The drawing under review shows one solid part. Ordinate dimensions are in mm from its lowest x, y, z. A direction names the side the tool comes from. Coordinates: 2 decimals unless noted, no trailing zeros. Loops run counter-clockwise (first coordinate to the right, second up) from the corner with the lowest first, then second, coordinate; pieces in that order, holes last. Notation, with made-up numbers: (51.5, -1.5) - (57.5, -1.5) arc R11 cw to (57.5, 2.5) - close; hole circle Ø3 at (45.5, -14). An arc over 180 degrees is marked (long way). Answer as a JSON object with one key per item and string values. Group by question number.
Item 1: Clearance check with flat-ended pins moving along their axes: pin 1 (3 mm diameter, centred on x = 10.5, y = 11.5, fed in from +Z); pin 2 (4 mm diameter, centred on x = 18.5, y = 15, fed in from +Z); pin 3 (3 mm diameter, centred on x = 13.5, y = 14, fed in from +Z). State where each tip first meets the part, or that it passes through.
Item 2: We need section D-D (x = 17.5). Give the boundary of the cut face in (y, z).
Item 3: Tool access review of the marked faces 1 and 2: name each direction out of +Z, -Z, +X, -X, +Y, -Y from which nothing blocks a thin tool from reaching the whole face with its end or side.
Item 4: Mouldability with a two-part tool opening along X and no side actions: class the marked faces 3, 4 and 5 as released by +X, released by -X, zero draft, split by the parting line, or undercut.
Item 5: We need section C-C (y = 11). Give the boundary of the cut face in (x, z).
Item 6: We need section A-A (z = 11). Give the boundary of the cut face in (x, y).
Item 7: We need section B-B (x = 11.75). Give the boundary of the cut face in (y, z), then the cut area to 3 significant figures.
Item 8: To check wall thickness, follow line 1 (Y direction, x = 12.5, z = 1.9); line 2 (X direction, y = 14.75, z = 2.75); line 3 (Y direction, x = 10.75, z = 4.5). State the ranges of each line that lie inside material, in increasing order.
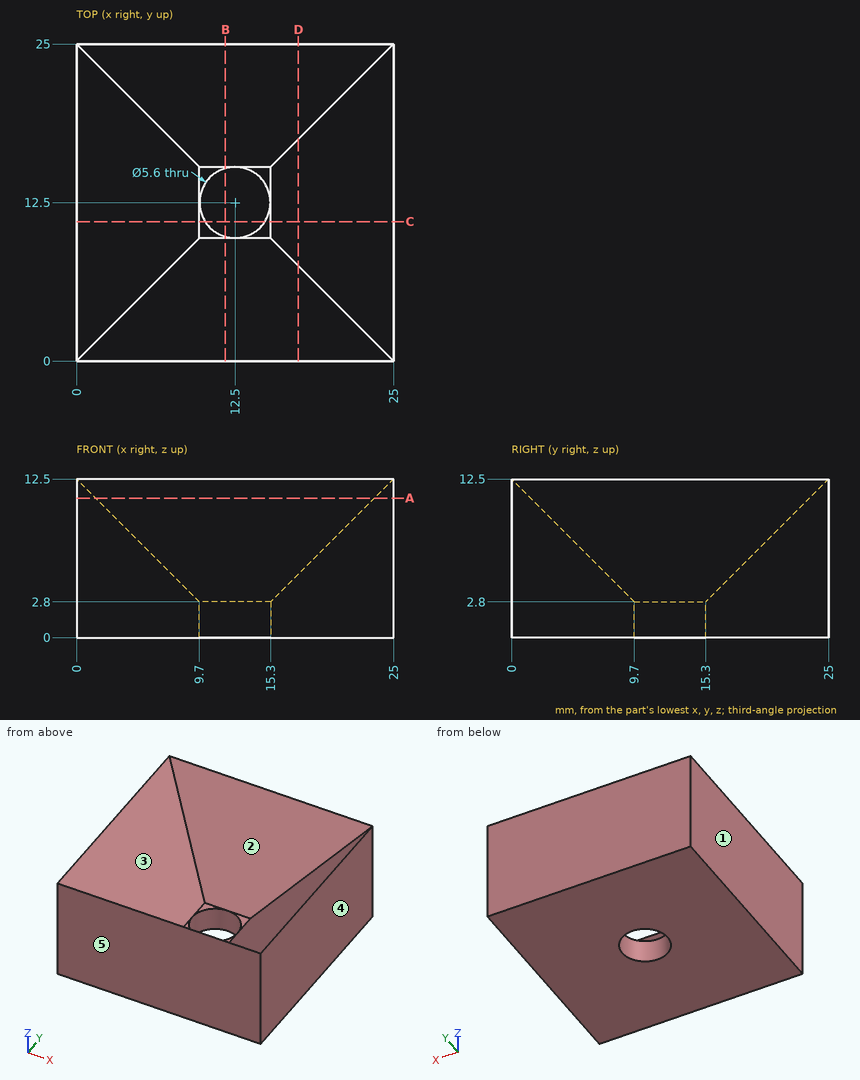
Check sheet entries:
{
 "1": {"pin 1": "stops at z = 3.5", "pin 2": "stops at z = 8", "pin 3": "stops at z = 3"},
 "2": {"outline": "(0, 0) - (25, 0) - (25, 12.5) - (17.5, 5) - (7.5, 5) - (0, 12.5) - close"},
 "3": {"face 1": "+Z, -Z, -X, +Y, -Y", "face 2": "+Z"},
 "4": {"face 3": "undercut", "face 4": "released by +X", "face 5": "zero draft"},
 "5": {"outline": "(0, 0) - (10.14, 0) - (10.14, 2.8) - (9.7, 2.8) - (0, 12.5) - close; (14.86, 0) - (25, 0) - (25, 12.5) - (15.3, 2.8) - (14.86, 2.8) - close"},
 "6": {"outline": "(0, 0) - (25, 0) - (25, 25) - (0, 25) - close; hole (1.5, 1.5) - (23.5, 1.5) - (23.5, 23.5) - (1.5, 23.5) - close"},
 "7": {"outline": "(0, 0) - (9.8, 0) - (9.8, 2.8) - (9.7, 2.8) - (0, 12.5) - close; (15.2, 0) - (25, 0) - (25, 12.5) - (15.3, 2.8) - (15.2, 2.8) - close", "area": "149 mm2"},
 "8": {"line 1": "y = 0 to 9.7, 15.3 to 25", "line 2": "x = 0 to 10.83, 14.17 to 25", "line 3": "y = 0 to 8, 17 to 25"}
}
